Part print with two shaded views. Sizes in mm from the minimum x, y, z corner. A direction names the side the tool comes from. Round coordinates to 2 decimals unless told otherwise and drop trailing zeros. Loops run counter-clockwise (first coordinate to the right, second up) from the corner with the lowest first, then second, coordinate; pieces in that order, holes last. Notation, with made-up numbers: M -3.5,86.5 L 49.5,86.5 A31 ccw 49.5,121.5 Z; hole C 12.5,81 d2. An arc over 180 degrees is marked long. Use a Markdown table: item, result. Add a question column.
Item 1: Wall check: L1, parallel to Y at x = 24.4, z = 11.85; L2, parallel to X at y = 12.5, z = 10.5; L3, parallel to Z at x = 30, y = 29. Give the ranges that are in metal, low to high. Write a range as from..to.
Item 2: Saw through at B-B on y = 16. Write the cut outline in (x, z).
Item 3: Two-plate mould, pull along Y, no slides. Class the marked faces 6, 7 and 8: +Y half, -Y half, draft (parallel to the pull), parting line (faces both ways), or undercut.
Item 4: Saw through at D-D on y = 9. Write the cut outline in (x, z).
Item 5: Saw through at C-C on z = 16.5. Write the cut outline in (x, y) (1 decimal).
Item 6: Saw through at A-A on z = 11.85. Write the cut outline in (x, y).
Item 7: Tool access for the marked faces 1, 2, 3, 4 and 5: list every direction of +Z, -Z, +X, -X, +Y, -Y with a clear straight run to the whole face (end or side of a thin tool).
Item 8: Pin check, flat tips, straight feed: P1, Ø5.5, axis at y = 18, z = 11.85, coming from the -X side; P2, Ø4.5, axis at x = 23, z = 8.5, coming from the +Y side; P3, Ø8, axis at x = 22.5, y = 11.5, coming from the +Z side; P4, Ø4.5, axis at x = 24, z = 10.5, coming from the -Y side. Stop position of each tip, or through.
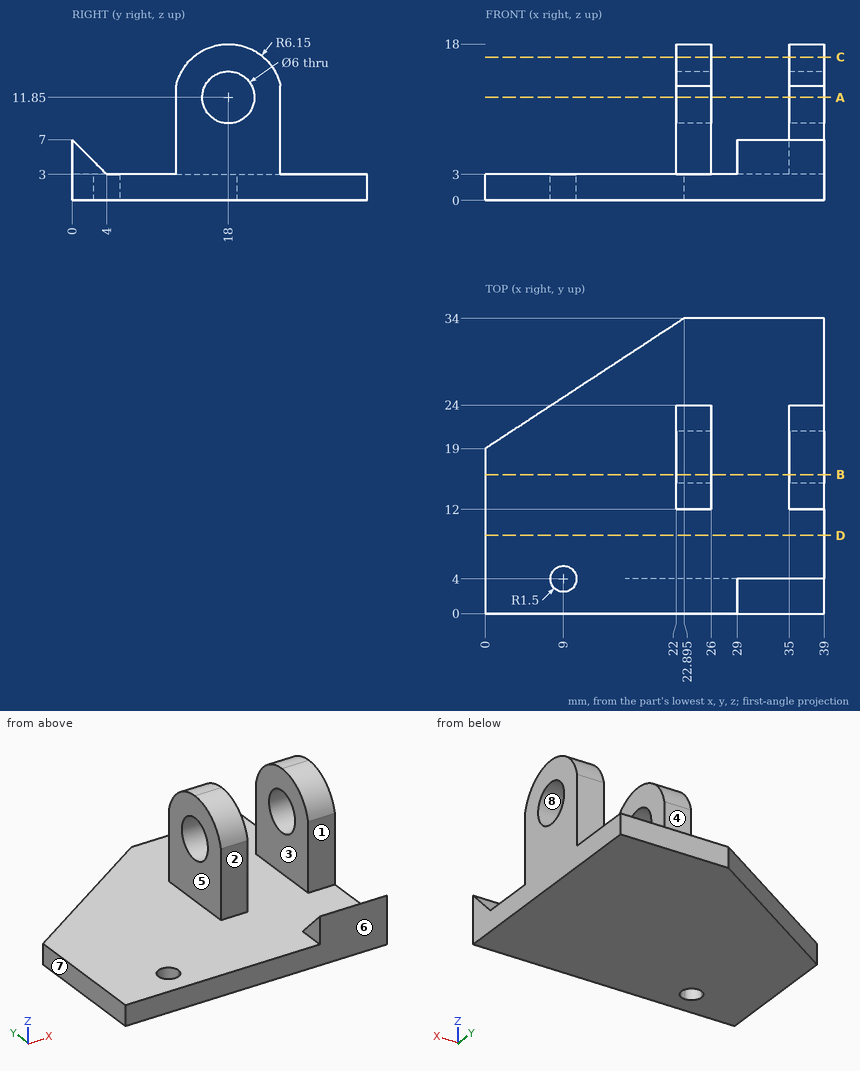
Entries:
| question | item | result |
|---|---|---|
| 1 | L1 | 12..15, 21..24 |
| 1 | L2 | 22..26, 35..39 |
| 1 | L3 | 0..3 |
| 2 | outline | M 0,0 L 39,0 L 39,9.61 L 35,9.61 L 35,3 L 26,3 L 26,9.61 L 22,9.61 L 22,3 L 0,3 Z; M 22,14.09 L 26,14.09 L 26,17.67 L 22,17.67 Z; M 35,14.09 L 39,14.09 L 39,17.67 L 35,17.67 Z |
| 3 | face 6 | -Y half |
| 3 | face 7 | draft |
| 3 | face 8 | undercut |
| 4 | outline | M 0,0 L 39,0 L 39,3 L 0,3 Z |
| 5 | outline | M 22,14 L 26,14 L 26,22 L 22,22 Z; M 35,14 L 39,14 L 39,22 L 35,22 Z |
| 6 | outline | M 22,12 L 26,12 L 26,15 L 22,15 Z; M 22,21 L 26,21 L 26,24 L 22,24 Z; M 35,12 L 39,12 L 39,15 L 35,15 Z; M 35,21 L 39,21 L 39,24 L 35,24 Z |
| 7 | face 1 | +Z, +X, -X |
| 7 | face 2 | +Z, +X, -X, -Y |
| 7 | face 3 | +Z, +Y |
| 7 | face 4 | +Z, +X, -X, +Y |
| 7 | face 5 | +Z, -X, +Y, -Y |
| 8 | P1 | through |
| 8 | P2 | y = 24 |
| 8 | P3 | z = 17.47 |
| 8 | P4 | y = 12 |
